Can you work these out from the drawing? Everything is in mm from the part's minimum corner. A direction names the side the tool comes from. Round coordinates to 2 decimals unless told otherwise and drop trailing zeros. Write each loop counter-clockwise with the first axis right and the second up, starting at its lowest first coordinate (ties: lowest second). Pieces come first, ordered by that corner, then holes. Notation, with made-up numbers: M 71,1 L 98,1 A25 cw 98,16 Z; hole C 28.25,-18.5 d4. An arc over 180 degrees is marked long. Answer in a Markdown table with one row per item. Add a question column.
(1) Suppose I cut it at D-D, the plane x = 27.5. Write out the boundary of the cut face in (y, z).
(2) For the marked faces 5 and 6, which set-ups out of +Z, -Z, +X, -X, +Y, -Y let a thin tool reach every point of the face, with its end or its side?
(3) I'm going to push flat-ended pins straight in: pin 1 (0.8 mm diameter, centred on y = 11.5, z = 9.5, fed in from +X); pin 2 (3 mm diameter, centred on y = 8.5, z = 7, fed in from +X); pin 3 (1 mm diameter, centred on y = 9.5, z = 2.5, fed in from +X). Where does each tip first touch, or does it pass through?
(4) Suppose I cut it at B-B, the plane y = 4. Write out the boundary of the cut face in (x, z).
(5) If we mould it in two halves opening along X, with no side actions, what happens to the marked faces 1, 2, 3 and 4? For each: released by +X, released by -X, zero draft, split by the parting line, or undercut.
(6) If I drill on probe 1 along Y at (x, z) = (16.5, 4.5); probe 2 along X at (y, z) = (5.5, 2.75); probe 3 along X at (y, z) = (2, 22), over which ranges is the centre line in solid material (lowest first)?
(7) Suppose I cut it at A-A, the plane x = 20.25. Write out the boundary of the cut face in (y, z), then the cut area to 3 significant figures.
(8) Suppose I cut it at C-C, the plane z = 17. Write out the boundary of the cut face in (x, y).
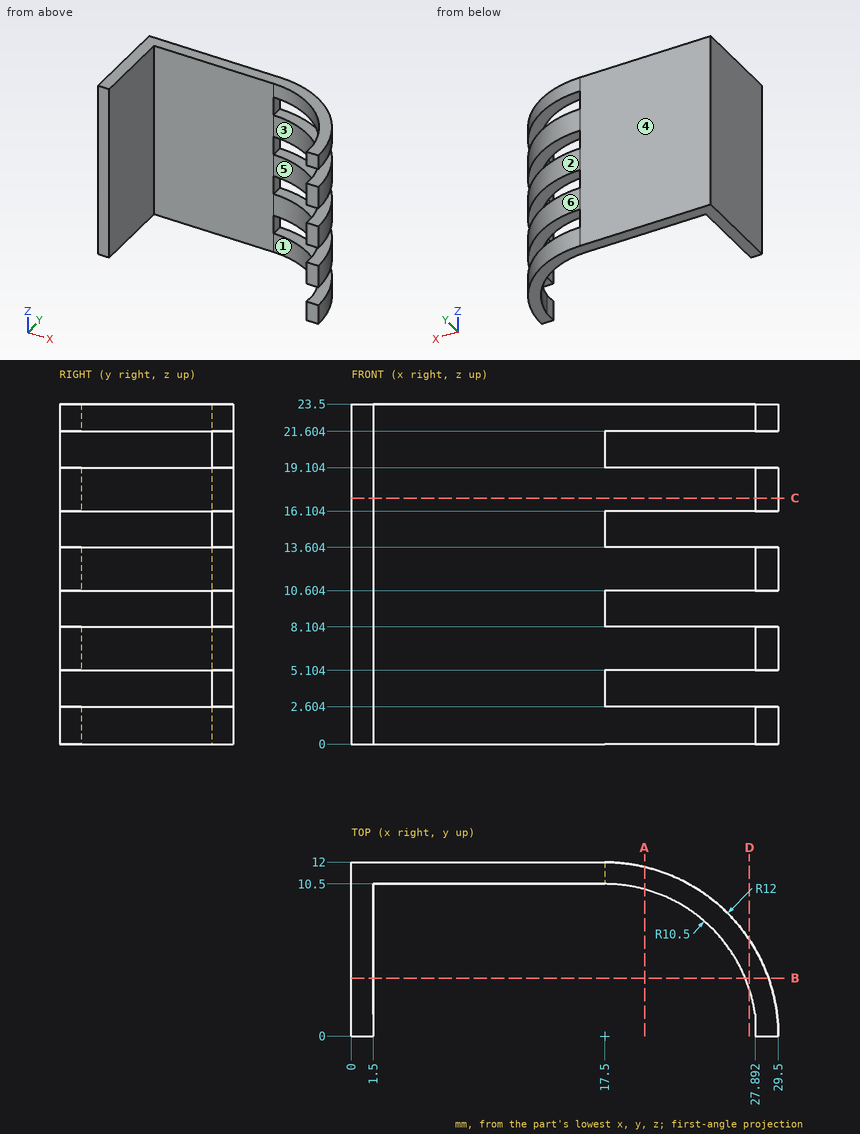
Calculated:
| question | item | result |
|---|---|---|
| 1 | outline | M 3.2,0 L 6.63,0 L 6.63,2.6 L 3.2,2.6 Z; M 3.2,5.1 L 6.63,5.1 L 6.63,8.1 L 3.2,8.1 Z; M 3.2,10.6 L 6.63,10.6 L 6.63,13.6 L 3.2,13.6 Z; M 3.2,16.1 L 6.63,16.1 L 6.63,19.1 L 3.2,19.1 Z; M 3.2,21.6 L 6.63,21.6 L 6.63,23.5 L 3.2,23.5 Z |
| 2 | face 5 | +Z, -Z, -Y |
| 2 | face 6 | +Z, -Z, +X, +Y |
| 3 | pin 1 | x = 17.5 |
| 3 | pin 2 | x = 27.25 |
| 3 | pin 3 | x = 25.44 |
| 4 | outline | M 0,0 L 1.5,0 L 1.5,23.5 L 0,23.5 Z; M 27.21,0 L 28.81,0 L 28.81,2.6 L 27.21,2.6 Z; M 27.21,5.1 L 28.81,5.1 L 28.81,8.1 L 27.21,8.1 Z; M 27.21,10.6 L 28.81,10.6 L 28.81,13.6 L 27.21,13.6 Z; M 27.21,16.1 L 28.81,16.1 L 28.81,19.1 L 27.21,19.1 Z; M 27.21,21.6 L 28.81,21.6 L 28.81,23.5 L 27.21,23.5 Z |
| 5 | face 1 | undercut |
| 5 | face 2 | released by +X |
| 5 | face 3 | undercut |
| 5 | face 4 | zero draft |
| 6 | probe 1 | 10.5 to 12 |
| 6 | probe 2 | 0 to 1.5 |
| 6 | probe 3 | 0 to 1.5, 27.81 to 29.33 |
| 7 | outline | M 10.13,0 L 11.68,0 L 11.68,2.6 L 10.13,2.6 Z; M 10.13,5.1 L 11.68,5.1 L 11.68,8.1 L 10.13,8.1 Z; M 10.13,10.6 L 11.68,10.6 L 11.68,13.6 L 10.13,13.6 Z; M 10.13,16.1 L 11.68,16.1 L 11.68,19.1 L 10.13,19.1 Z; M 10.13,21.6 L 11.68,21.6 L 11.68,23.5 L 10.13,23.5 Z |
| 7 | area | 20.9 mm² |
| 8 | outline | M 0,0 L 1.5,0 L 1.5,10.5 L 17.5,10.5 A10.5 cw 27.89,1.5 L 27.89,0 L 29.5,0 A12 ccw 17.5,12 L 0,12 Z |
